```python
from build123d import *

# Parameters (mm, degrees)
F0_W     = 142
F0_H     = 62
F1_DEPTH = 50
F2_W     = 138
F2_H     = 58
F3_DEPTH = 48
F6_W     = 40
F6_H     = 30
F7_DEPTH = 2
F8_W     = 2
F8_H     = 33
F9_DEPTH = 25


# Not quite as in the source:
# - a feature names something its author has since deleted; it is built from what else it names


with BuildPart() as f1:
    # F0 (on Top) → F1 (new body)
    with BuildSketch(Plane.XY):
        with Locations((34.9231133461, -3.5940962459)):
            Rectangle(F0_W, F0_H)
    extrude(amount=F1_DEPTH)

    # F2 (on face) → F3 (cut)
    with BuildSketch(Plane.XY.offset(50)):
        with Locations((34.9231133461, -3.5940962459)):
            Rectangle(F2_W, F2_H)
    extrude(amount=-F3_DEPTH, mode=Mode.SUBTRACT)

    # F6 (on face) → F7 (cut)
    with BuildSketch(Plane.XZ.offset(34.5940962459)):
        with Locations((83.9231133461, 17)):
            Rectangle(F6_W, F6_H)
    extrude(amount=-F7_DEPTH, mode=Mode.SUBTRACT)

    # F8 (on face) → F9 (join)
    with BuildSketch(Plane.XY.offset(2)):
        with Locations((61.7997199297, -16.0940962459)):
            Rectangle(F8_W, F8_H)
    extrude(amount=F9_DEPTH)


solid = f1.part
```
Work out the finished part from the listing and answer in its coordinate system (mm). A direction names the side the tool comes from. Give positions to 0.01 mm unless a question says otherwise; leave off trailing zeros. Order: outer loops, then holes, each group sorted by start corner. A loop starts at its lowest first (then second) coordinate and runs counter-clockwise, first axis right, second up. Notation, with made-up numbers: M 11,42.5 L 50,42.5 A10 cw 50,60.5 Z; hole C 9,57.25 d5. An arc over 180 degrees is marked long. Return JSON: item names as keys, results as strings.
1) Section B-B, the plane z = 42 is taken. Write down the section's boundary in (x, y).
Resolved:
{"outline": "M -36.08,-34.59 L 105.92,-34.59 L 105.92,27.41 L -36.08,27.41 Z; hole M -34.08,-32.59 L 103.92,-32.59 L 103.92,25.41 L -34.08,25.41 Z"}
2) Section C-C, the plane y = -21 is taken. Write down the section's boundary in (x, z), plus the area to 3 significant figures.
Resolved:
{"outline": "M -36.08,0 L 105.92,0 L 105.92,50 L 103.92,50 L 103.92,2 L 62.8,2 L 62.8,27 L 60.8,27 L 60.8,2 L -34.08,2 L -34.08,50 L -36.08,50 Z", "area": "526 mm^2"}
3) Section D-D, the plane z = 7.5 is taken. Write down the section's boundary in (x, y), plus the area to 3 significant figures.
Resolved:
{"outline": "M -36.08,-34.59 L 63.92,-34.59 L 63.92,-32.59 L 62.8,-32.59 L 62.8,0.41 L 60.8,0.41 L 60.8,-32.59 L -34.08,-32.59 L -34.08,25.41 L 103.92,25.41 L 103.92,-34.59 L 105.92,-34.59 L 105.92,27.41 L -36.08,27.41 Z", "area": "786 mm^2"}
4) A tool of negligible diameter and unlimited length cuts with its end or side. For faces 4 (the flat face through (105.923, -4, 25)), 5 (the flat face through (34, 25.406, 26)), from which of +Z, -Z, +X, -X, +Y, -Y can it reach the whole face along a straight path? Write none if from no direction.
Resolved:
{"face 4": "+Z, -Z, +X, +Y, -Y", "face 5": "+Z"}
5) For a pull along X with two mould halves and no side action, classify faces 1 (the flat face through (60.8, -16, 14)), 2 (the flat face through (35, -33, 50)), 3 (the flat face through (-36.077, -4, 25)) as +X half, -X half, draft (parallel to the pull), parting line (faces both ways), or undercut.
Resolved:
{"face 1": "undercut", "face 2": "draft", "face 3": "-X half"}
6) Straight lines are drawn through the part: line 1 along X through (y, z) = (-12, 22.5); line 2 along X through (y, z) = (17, 15.5); line 3 along Y through (x, z) = (34, 39.5). For each, find the intervals that lie inside material, in ascending order. Write a range as [from, to].
Resolved:
{"line 1": "[-36.08, -34.08], [60.8, 62.8], [103.92, 105.92]", "line 2": "[-36.08, -34.08], [103.92, 105.92]", "line 3": "[-34.59, -32.59], [25.41, 27.41]"}
7) Section A-A, the plane x = 93 is taken. Write down the section's boundary in (y, z).
Resolved:
{"outline": "M -34.59,0 L 27.41,0 L 27.41,50 L 25.41,50 L 25.41,2 L -34.59,2 Z; M -34.59,32 L -32.59,32 L -32.59,50 L -34.59,50 Z"}
8) Each of these flat-tipped pins is pushed along its axis until it touches: pin 1 (10 mm diameter, centred on x = -21, y = -18.5, fed in from -Z); pin 2 (8 mm diameter, centred on x = 12, y = -15, fed in from +Z); pin 3 (1 mm diameter, centred on x = 62, y = -18, fed in from +Z). Where does it stop, or does it pass through?
Resolved:
{"pin 1": "z = 0", "pin 2": "z = 2", "pin 3": "z = 27"}
